Work out the finished part from the listing and answer in its coordinate system (mm). Round coordinates to 2 decimals unless told otherwise and drop trailing zeros. Loops run counter-clockwise (first coordinate to the right, second up) from the corner with the lowest first, then second, coordinate; pieces in that order, holes last. Notation, with made-up numbers: M 47.5,68.5 L 75.5,68.5 A26 cw 75.5,104.5 Z; hole C -10.5,26.5 d10. An arc over 180 degrees is marked long. One line per item, written item: value.
```python
from build123d import *

# Parameters (mm, degrees)
F0_W      = 40
F0_H      = 250
F1_DEPTH  = 200
F4_R      = 5
F5_DEPTH  = 20
F3_R      = 5
F6_DEPTH  = 20
F7_R      = 5
F8_DEPTH  = 20
F9_R      = 5
F10_DEPTH = 20
F11_R     = 5
F12_DEPTH = 20
F13_R     = 5
F14_DEPTH = 20


with BuildPart() as f1:
    # F0 (on Right) → F1 (new body, symmetric)
    with BuildSketch(Plane.YZ):
        with Locations((20, 125)):
            Rectangle(F0_W, F0_H)
    extrude(amount=F1_DEPTH, both=True)

    # F4 (on face) → F5 (cut)
    with BuildSketch(Plane.XZ):
        with Locations((-79.978161, 100)):
            Circle(F4_R)
    extrude(amount=-F5_DEPTH, mode=Mode.SUBTRACT)

    # F3 (on face) → F6 (cut)
    with BuildSketch(Plane.XZ):
        with Locations((-79.879753, 150)):
            Circle(F3_R)
    extrude(amount=-F6_DEPTH, mode=Mode.SUBTRACT)

    # F7 (on face) → F8 (cut)
    with BuildSketch(Plane.XY.offset(250)):
        with Locations((-165, 20)):
            Circle(F7_R)
    extrude(amount=-F8_DEPTH, mode=Mode.SUBTRACT)

    # F9 (on face) → F10 (cut)
    with BuildSketch(Plane.XY.offset(250)):
        with Locations((165, 20)):
            Circle(F9_R)
    extrude(amount=-F10_DEPTH, mode=Mode.SUBTRACT)

    # F11 (on face) → F12 (cut)
    with BuildSketch(Plane(origin=(0, 0, 0), x_dir=(1, 0, 0), z_dir=(0, 0, -1))):
        with Locations((-165, -20)):
            Circle(F11_R)
    extrude(amount=-F12_DEPTH, mode=Mode.SUBTRACT)

    # F13 (on face) → F14 (cut)
    with BuildSketch(Plane(origin=(0, 0, 0), x_dir=(1, 0, 0), z_dir=(0, 0, -1))):
        with Locations((165, -20)):
            Circle(F13_R)
    extrude(amount=-F14_DEPTH, mode=Mode.SUBTRACT)


solid = f1.part
```
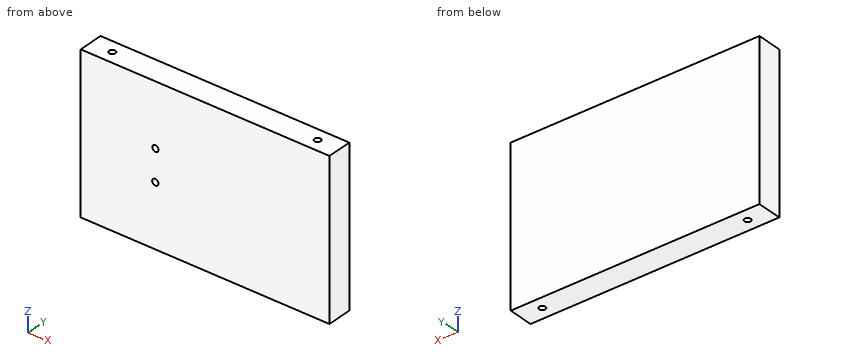
1) Find section A-A (x = -165). Give the vertices of the cut face in (y, z).
Check values:
outline: M 0,0 L 15,0 L 15,20 L 25,20 L 25,0 L 40,0 L 40,250 L 25,250 L 25,230 L 15,230 L 15,250 L 0,250 Z
2) Each of these flat-tipped pins is pushed along its axis until it touches: pin 1 (8 mm diameter, centred on x = 165, y = 20, fed in from -Z); pin 2 (3 mm diameter, centred on x = -167, y = 18.5, fed in from +Z); pin 3 (3 mm diameter, centred on x = -77.5, z = 99, fed in from -Y). Where does it stop, or does it pass through?
Check values:
pin 1: z = 20
pin 2: z = 230
pin 3: y = 20
3) Find the intervals of material crossed by probe 1 along Y at (x, z) = (165, 237.5); probe 2 along X at (y, z) = (20, 9.5), in increasing order. Write a range as from..to.
Check values:
probe 1: 0..15, 25..40
probe 2: -200..-170, -160..160, 170..200
